Design review of the part built by this model. Coordinates are the model's own, in mm. A direction names the side the tool comes from. Round coordinates to 2 decimals unless told otherwise and drop trailing zeros. Write each loop counter-clockwise with the first axis right and the second up, starting at its lowest first coordinate (ties: lowest second). Pieces come first, ordered by that corner, then holes. Notation, with made-up numbers: M 6.25,59 L 54.25,59 A18 cw 54.25,72 Z; hole C -2,7 d8. An arc over 180 degrees is marked long. Use CSV: the item, a comma, the result in double quotes.
from build123d import *

# Parameters (mm, degrees)
SKETCH1_W                 = 29
SKETCH1_H                 = 29
BOSS_EXTRUDE1_DEPTH       = 15
SKETCH2_R                 = 14.5
BOSS_EXTRUDE2_DEPTH       = 7.274
M2X0_4_TAPPED_HOLE1_D     = 1.6
M2X0_4_TAPPED_HOLE1_DEPTH = 2.5
M2X0_4_TAPPED_HOLE1_TIP   = 0.480688495
M2X0_4_TAPPED_HOLE2_D     = 1.6
M2X0_4_TAPPED_HOLE2_DEPTH = 2
M2X0_4_TAPPED_HOLE2_TIP   = 0.480688495
M2X0_4_TAPPED_HOLE3_D     = 1.6
M2X0_4_TAPPED_HOLE3_DEPTH = 2.5
M2X0_4_TAPPED_HOLE3_TIP   = 0.480688495
M3X0_5_TAPPED_HOLE2_D     = 2.5
M3X0_5_TAPPED_HOLE2_DEPTH = 2.8
M3X0_5_TAPPED_HOLE2_TIP   = 0.751075774
M3X0_5_TAPPED_HOLE1_D     = 2.5
M3X0_5_TAPPED_HOLE1_DEPTH = 2.5
M3X0_5_TAPPED_HOLE1_TIP   = 0.751075774
SKETCH10_R                = 4.4
BOSS_EXTRUDE3_DEPTH       = 6.5


with BuildPart() as part:
    # Sketch1 → Boss-Extrude1 (new body, symmetric)
    with BuildSketch(Plane.XY):
        Rectangle(SKETCH1_W, SKETCH1_H)
    extrude(amount=BOSS_EXTRUDE1_DEPTH, both=True)

    # Sketch2 → Boss-Extrude2 (add)
    with BuildSketch(Plane.XY.offset(15)):
        Circle(SKETCH2_R)
    extrude(amount=BOSS_EXTRUDE2_DEPTH)

    # M2x0.4 Tapped Hole1
    with Locations(Plane(origin=(-6, 14.5, 13), x_dir=(0, 0, 1), z_dir=(0, 1, 0))):
        with Locations((0, 0), (0, 12)):
            Hole(M2X0_4_TAPPED_HOLE1_D / 2, depth=M2X0_4_TAPPED_HOLE1_DEPTH)
            with Locations((0, 0, -(M2X0_4_TAPPED_HOLE1_DEPTH + M2X0_4_TAPPED_HOLE1_TIP / 2))):  # 118° drill point
                Cone(0, M2X0_4_TAPPED_HOLE1_D / 2, M2X0_4_TAPPED_HOLE1_TIP, mode=Mode.SUBTRACT)

    # M2x0.4 Tapped Hole2
    with Locations(Plane(origin=(-6, -14.5, -11.7), x_dir=(0, 0, -1), z_dir=(0, -1, 0))):
        with Locations((0, 0), (0, 12)):
            Hole(M2X0_4_TAPPED_HOLE2_D / 2, depth=M2X0_4_TAPPED_HOLE2_DEPTH)
            with Locations((0, 0, -(M2X0_4_TAPPED_HOLE2_DEPTH + M2X0_4_TAPPED_HOLE2_TIP / 2))):  # 118° drill point
                Cone(0, M2X0_4_TAPPED_HOLE2_D / 2, M2X0_4_TAPPED_HOLE2_TIP, mode=Mode.SUBTRACT)

    # M2x0.4 Tapped Hole3
    with Locations(Plane(origin=(-6, -14.5, 10.5), x_dir=(0, 0, -1), z_dir=(0, -1, 0))):
        with Locations((0, 0), (0, 12)):
            Hole(M2X0_4_TAPPED_HOLE3_D / 2, depth=M2X0_4_TAPPED_HOLE3_DEPTH)
            with Locations((0, 0, -(M2X0_4_TAPPED_HOLE3_DEPTH + M2X0_4_TAPPED_HOLE3_TIP / 2))):  # 118° drill point
                Cone(0, M2X0_4_TAPPED_HOLE3_D / 2, M2X0_4_TAPPED_HOLE3_TIP, mode=Mode.SUBTRACT)

    # M3x0.5 Tapped Hole2
    with Locations(Plane(origin=(10, -14.5, 12), x_dir=(0, 0, -1), z_dir=(0, -1, 0))):
        with Locations((0, 0), (0, -20)):
            Hole(M3X0_5_TAPPED_HOLE2_D / 2, depth=M3X0_5_TAPPED_HOLE2_DEPTH)
            with Locations((0, 0, -(M3X0_5_TAPPED_HOLE2_DEPTH + M3X0_5_TAPPED_HOLE2_TIP / 2))):  # 118° drill point
                Cone(0, M3X0_5_TAPPED_HOLE2_D / 2, M3X0_5_TAPPED_HOLE2_TIP, mode=Mode.SUBTRACT)

    # M3x0.5 Tapped Hole1
    with Locations(Plane(origin=(0, -14.5, -11.7), x_dir=(0, 0, -1), z_dir=(0, -1, 0))):
        with Locations((0, 0)):
            Hole(M3X0_5_TAPPED_HOLE1_D / 2, depth=M3X0_5_TAPPED_HOLE1_DEPTH)
            with Locations((0, 0, -(M3X0_5_TAPPED_HOLE1_DEPTH + M3X0_5_TAPPED_HOLE1_TIP / 2))):  # 118° drill point
                Cone(0, M3X0_5_TAPPED_HOLE1_D / 2, M3X0_5_TAPPED_HOLE1_TIP, mode=Mode.SUBTRACT)

    # Sketch10 → Boss-Extrude3 (add)
    with BuildSketch(Plane(origin=(0, 0, -15), x_dir=(-1, 0, 0), z_dir=(0, 0, -1))):
        with Locations((-6.5, 9)):
            Circle(SKETCH10_R)
    extrude(amount=BOSS_EXTRUDE3_DEPTH)


solid = part.part
1) Add section A-A on y = -7. Write out the cut boundary in (x, z), then the cut area to 3 significant figures.
Answers:
outline,"M -14.5,-15 L 14.5,-15 L 14.5,15 L 12.7,15 L 12.7,22.27 L -12.7,22.27 L -12.7,15 L -14.5,15 Z"
area,"1,050 mm²"
2) The part is to be moulded in two halves that separate along X. For faces 1 (the face through (0, 14.5, 0)), 2 (the face through (6.006, -11.603, 10.639)), 3 (the face through (6.54, -13.23, 9.91)), 4 (the face through (6.691, -12.864, 18.586)), say which applies: released by +X, released by -X, zero draft, split by the parting line, or undercut.
Answers:
face 1,"zero draft"
face 2,"undercut"
face 3,"undercut"
face 4,"split by the parting line"
3) For pin 1 Ø1 at (x, z) = (-6, 10.5) entering from -Y; pin 2 Ø1.4 at (x, z) = (6, -11.7) entering from -Y; pin 3 Ø3 at (x, z) = (-7.5, 17) entering from -Y, all flat-tipped, find the tip position at first contact; note any pin that passes through.
Answers:
pin 1,"y = -11.82"
pin 2,"y = -12.44"
pin 3,"y = -13.2"
4) Machinability: for faces 5 (the face through (12, -12, 15)), 6 (the face through (-12, 11, 15)), 7 (the face through (6.793, -13.486, -11.804)), which of the approach directions +Z, -Z, +X, -X, +Y, -Y give a long, thin tool a straight path to every point of the face, cutting with its end or side? Answer none if there is none.
Answers:
face 5,"+Z, +X, -Y"
face 6,"+Z, -X, +Y"
face 7,"-Y"
5) Add section B-B on y = 9. Write out the cut boundary in (x, z).
Answers:
outline,"M -14.5,-15 L 2.1,-15 L 2.1,-21.5 L 10.9,-21.5 L 10.9,-15 L 14.5,-15 L 14.5,15 L 11.37,15 L 11.37,22.27 L -11.37,22.27 L -11.37,15 L -14.5,15 Z"
6) Wall thickness on line 1 along X through (y, z) = (-13.85, 12); line 2 along X through (y, z) = (12.65, 13); line 3 along Z through (x, y) = (-6, -13.05): over which ranges is each line inside the solid? List them lowest first. Write a range as [from, to].
Answers:
line 1,"[-14.5, -11.25], [-8.75, 8.75], [11.25, 14.5]"
line 2,"[-14.5, -6.8], [-5.2, 5.2], [6.8, 14.5]"
line 3,"[-15, -12.5], [-10.9, 9.7], [11.3, 22.27]"
